Geometry: final body of the model. Coordinates: model frame, mm. A direction names the side the tool comes from. Give positions to 0.01 mm unless a question says otherwise; leave off trailing zeros. Write each loop counter-clockwise with the first axis right and the second up, starting at its lowest first coordinate (ties: lowest second). Pieces come first, ordered by that corner, then holes.
Q1. Mould query, pull axis Y, two halves, no side actions, for faces 4 (the flat face through (15.912, 5, 49)), 5 (the flat face through (-13, 19.546, 49)), 6 (the flat face through (-5.338, 7, 49)), 7 (the flat face through (-9, -4.704, 49)). Classes: +Y half, -Y half, draft (parallel to the pull), parting line (faces both ways), or undercut.
Q2. Section B-B (y = -13). Return the cut outline in (x, z).
Q3. Section A-A (y = 2). Return the cut outline in (x, z).
Q4. Section D-D (z = 79.5). State how many separate pieces and enclosed holes the cut face has, plus the area to 3 significant figures.
Q5. Line query: line 1 (Y direction, x = 5, z = 38.5); line 2 (Y direction, x = -15, z = 9); line 3 (X direction, y = 4, z = 45). Output: solid intervals per line, ascending.
Q6. Section C-C (x = -13). Return the cut outline in (y, z).
Q7. Pin query (flat end, axial travel): pin 1 Ø8 at (x, z) = (-4.5, 67) entering from +Y; pin 2 Ø4 at (y, z) = (0.5, 32) entering from -X; pin 3 Ø1 at (x, y) = (8, -4) entering from -Z. Return the tip coordinate at first contact, or that it passes through.
Q8. Reachability of faces 1 (the flat face through (17, -4.704, 49)), 2 (the flat face through (-10.088, -6, 49)), 3 (the flat face through (-1, -6.454, 49)) from +Z, -Z, +X, -X, +Y, -Y: full face, straight path, thin tool, end or side. Return the list, or none.
from build123d import *

# Parameters (mm, degrees)
SKETCH_1_R      = 3.9
SKETCH_1_R_2    = 3.4
EXTRUDE_1_DEPTH = 100


with BuildPart() as part:
    # 草图1 → 凸台-拉伸1 (new body)
    with BuildSketch(Plane.XY):
        Polygon((-5.338418149, 19.545792426), (-21.088418149, 19.545792426), (-21.088418149, 3.795792426), (-18.088418149, 3.795792426), (-18.088418149, 6.745792426), (-10.088418149, 6.745792426), (-10.088418149, 3.795792426), (-7.088418149, 3.795792426), (-7.088418149, -4.704207574), (-10.088418149, -4.704207574), (-10.088418149, -7.654207574), (-18.088418149, -7.654207574), (-18.088418149, -4.704207574), (-21.088418149, -4.704207574), (-21.088418149, -20.454207574), (-5.338418149, -20.454207574), (-5.338418149, -17.454207574), (-8.288418149, -17.454207574), (-8.288418149, -9.454207574), (-5.338418149, -9.454207574), (-5.338418149, -6.454207574), (3.161581851, -6.454207574), (3.161581851, -9.454207574), (6.111581851, -9.454207574), (6.111581851, -17.454207574), (3.161581851, -17.454207574), (3.161581851, -20.454207574), (18.911581851, -20.454207574), (18.911581851, -4.704207574), (15.911581851, -4.704207574), (15.911581851, -7.654207574), (7.911581851, -7.654207574), (7.911581851, -4.704207574), (4.911581851, -4.704207574), (4.911581851, 3.795792426), (7.911581851, 3.795792426), (7.911581851, 6.745792426), (15.911581851, 6.745792426), (15.911581851, 3.795792426), (18.911581851, 3.795792426), (18.911581851, 19.545792426), (3.161581851, 19.545792426), (3.161581851, 16.545792426), (6.111581851, 16.545792426), (6.111581851, 8.545792426), (3.161581851, 8.545792426), (3.161581851, 5.545792426), (-5.338418149, 5.545792426), (-5.338418149, 8.545792426), (-8.288418149, 8.545792426), (-8.288418149, 16.545792426), (-5.338418149, 16.545792426), align=None)
        with Locations((-14.688418149, 13.145792426)):
            Circle(SKETCH_1_R, mode=Mode.SUBTRACT)
        with Locations((12.511581851, 13.145792426)):
            Circle(SKETCH_1_R, mode=Mode.SUBTRACT)
        with Locations((-14.688418149, -14.054207574)):
            Circle(SKETCH_1_R, mode=Mode.SUBTRACT)
        with Locations((12.511581851, -14.054207574)):
            Circle(SKETCH_1_R, mode=Mode.SUBTRACT)
        with Locations((-1.088418149, -0.454207574)):
            Circle(SKETCH_1_R_2, mode=Mode.SUBTRACT)
    extrude(amount=EXTRUDE_1_DEPTH)


solid = part.part
Computed:
1. face 4: undercut
1. face 5: +Y half
1. face 6: draft
1. face 7: undercut
2. outline: (-21.09, 0) - (-18.44, 0) - (-18.44, 100) - (-21.09, 100) - close; (-10.93, 0) - (-8.29, 0) - (-8.29, 100) - (-10.93, 100) - close; (6.11, 0) - (8.76, 0) - (8.76, 100) - (6.11, 100) - close; (16.27, 0) - (18.91, 0) - (18.91, 100) - (16.27, 100) - close
3. outline: (-7.09, 0) - (-3.44, 0) - (-3.44, 100) - (-7.09, 100) - close; (1.26, 0) - (4.91, 0) - (4.91, 100) - (1.26, 100) - close
4. separate pieces: 1
4. enclosed holes: 5
4. area: 708 mm2
5. line 1: y = -20.45 to -17.45, -9.45 to -4.7, 3.8 to 8.55, 16.55 to 19.55
5. line 2: y = -20.45 to -17.94, -10.17 to -7.65, 6.75 to 9.26, 17.03 to 19.55
5. line 3: x = -21.09 to -18.09, -10.09 to 7.91, 15.91 to 18.91
6. outline: (-20.45, 0) - (-17.57, 0) - (-17.57, 100) - (-20.45, 100) - close; (-10.54, 0) - (-7.65, 0) - (-7.65, 100) - (-10.54, 100) - close; (6.75, 0) - (9.63, 0) - (9.63, 100) - (6.75, 100) - close; (16.66, 0) - (19.55, 0) - (19.55, 100) - (16.66, 100) - close
7. pin 1: stops at y = 19.55
7. pin 2: stops at x = -7.09
7. pin 3: passes through
8. face 1: +Z, -Z, +X
8. face 2: +Z, -Z
8. face 3: +Z, -Z, -Y
